Input: part model. Units: mm. Frame: model coordinates. Face numbers are marked on the shaded views. Give positions to 0.01 mm unless a question says otherwise; leave off trailing zeros. Write each loop counter-clockwise with the first axis right and the second up, starting at its lowest first coordinate (ties: lowest second). Pieces come first, ordered by that corner, then holes. Notation, with made-up numbers: (45.25, -10.5) - (54.25, -10.5) arc R12 ccw to (54.25, 6.5) - close; hole circle Ø7 at (83.5, 70). An arc over 180 degrees is marked (long way). Answer as CSV lines item,"result". Start each with the question number.
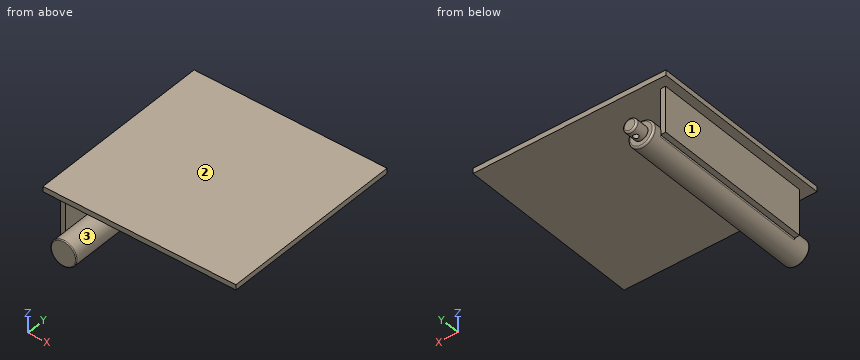
from build123d import *

# Parameters (mm, degrees)
SKETCH_1_W               = 110
SKETCH_1_H               = 106
EXTRUDE_1_DEPTH          = 3
SKETCH_2_W               = 3
SKETCH_2_H               = 94
EXTRUDE_2_DEPTH          = 38
EXTRUDE_3_DEPTH          = 5
EXTRUDE_3_DEPTH_BACK     = 104.122011
SKETCH_4_R               = 7.35
SKETCH_5_R               = 3.95
EXTRUDE_4_DEPTH          = 8
FILLET_2_R               = 1
CUT_EXTRUDE_1_DEPTH      = 155.044806793
CUT_EXTRUDE_1_DEPTH_BACK = 155.044806793
SKETCH_9_R               = 1.5
FILLET_3_R               = 0.5
SKETCH_11_W              = 3
SKETCH_11_H              = 94
CUT_EXTRUDE_3_DEPTH      = 12


with BuildPart() as part:
    # 草图1 → 凸台-拉伸1 (new body)
    with BuildSketch(Plane.XY):
        with Locations((55, 43)):
            Rectangle(SKETCH_1_W, SKETCH_1_H)
    extrude(amount=EXTRUDE_1_DEPTH)

    # 草图2 → 凸台-拉伸2 (add)
    with BuildSketch(Plane(origin=(0, 0, 0), x_dir=(-1, 0, 0), z_dir=(0, 0, -1))):
        with Locations((-6.5, 43)):
            Rectangle(SKETCH_2_W, SKETCH_2_H)
    extrude(amount=EXTRUDE_2_DEPTH)

    # 草图4 → 凸台-拉伸3 (add, two sides: drawn at the far end of the back side and taken through both)
    with BuildSketch(Plane(origin=(0, 90, 0), x_dir=(1, 0, 0), z_dir=(0, 1, 0)).offset(-EXTRUDE_3_DEPTH_BACK)):
        with Locations(Location((15, 25, 0), (0, 0, 270))):
            Circle(SKETCH_4_R)
    extrude(amount=EXTRUDE_3_DEPTH + EXTRUDE_3_DEPTH_BACK)

    # 草图5 → 凸台-拉伸4 (add)
    with BuildSketch(Plane(origin=(0, 95, 0), x_dir=(1, 0, 0), z_dir=(0, 1, 0))):
        with Locations(Location((15, 25, 0), (0, 0, 270))):
            Circle(SKETCH_5_R)
    extrude(amount=EXTRUDE_4_DEPTH)

    # 圆角2
    fillet_2_edges = [part.edges().sort_by_distance(p)[0] for p in [
        (15, 95, -32.35),
        (15, 103, -28.95),
    ]]
    fillet(fillet_2_edges, radius=FILLET_2_R)

    # 草图9 → 切除-拉伸1 (cut, two sides: drawn at the far end of the back side and taken through both)
    with BuildSketch(Plane(origin=(0, 0, -28.95), x_dir=(-1, 0, 0), z_dir=(0, 0, -1)).offset(-CUT_EXTRUDE_1_DEPTH_BACK)):
        with Locations(Location((-15, 98.677988735, 0), (0, 0, 90.000000013))):
            Circle(SKETCH_9_R)
    extrude(amount=CUT_EXTRUDE_1_DEPTH + CUT_EXTRUDE_1_DEPTH_BACK, mode=Mode.SUBTRACT)

    # 圆角3
    fillet_3_edges = [part.edges().sort_by_distance(p)[0] for p in [
        (15, -14.122011, -32.35),
    ]]
    fillet(fillet_3_edges, radius=FILLET_3_R)

    # 草图11 → 切除-拉伸3 (cut)
    with BuildSketch(Plane(origin=(0, 0, -38), x_dir=(-1, 0, 0), z_dir=(0, 0, -1))):
        with Locations((-6.5, 43)):
            Rectangle(SKETCH_11_W, SKETCH_11_H)
    extrude(amount=-CUT_EXTRUDE_3_DEPTH, mode=Mode.SUBTRACT)


solid = part.part
1) Contact query for flat-ended pins moving along their axis: P1, Ø1, axis at x = 68.5, y = 43.5, coming from the -Z side; P2, Ø1.5, axis at y = 2.5, z = -23.5, coming from the +X side; P3, Ø1.5, axis at x = 7, y = 36, coming from the -Z side. Output: stop coordinate, or through.
2) Cut plane B-B on y = 30. Output: boundary loops of the cut face in (x, z).
3) Pull-direction query (Z, two-part tool) for the marked faces 1, 2 and 3; classes: +Z half, -Z half, draft (parallel to the pull), parting line (faces both ways), or undercut.
4) Cut plane C-C on z = -10. Output: boundary loops of the cut face in (x, y), and give its area (3 significant figures).
5) Material intervals for line 1 (Z direction, x = 38.5, y = 72.5); line 2 (Z direction, x = 18.5, y = 94); line 3 (X direction, y = 85, z = -4), sorted ascending. Write a range as from..to.
6) Cut plane D-D on x = 90. Output: boundary loops of the cut face in (y, z).
7) Cut plane A-A on x = 15. Output: boundary loops of the cut face in (y, z), and give its area (3 significant figures).
Numbers:
1,P1,"stops at z = 0"
1,P2,"stops at x = 22.31"
1,P3,"stops at z = -26"
2,outline,"(0, 0) - (5, 0) - (5, -26) - (8, -26) - (8, -27.24) arc R7.35 ccw (long way) to (8, -22.76) - (8, 0) - (110, 0) - (110, 3) - (0, 3) - close"
3,face 1,"draft"
3,face 2,"+Z half"
3,face 3,"undercut"
4,outline,"(5, -4) - (8, -4) - (8, 90) - (5, 90) - close"
4,area,"282 mm²"
5,line 1,"z = 0..3"
5,line 2,"z = -31.46..-18.54, 0..3"
5,line 3,"x = 5..8"
6,outline,"(-10, 0) - (96, 0) - (96, 3) - (-10, 3) - close"
7,outline,"(-14.12, -31.85) arc R0.5 ccw to (-13.62, -32.35) - (94, -32.35) arc R1 ccw to (95, -31.35) - (95, -28.95) - (97.18, -28.95) - (97.18, -21.05) - (95, -21.05) - (95, -18.65) arc R1 ccw to (94, -17.65) - (-13.62, -17.65) arc R0.5 ccw to (-14.12, -18.15) - close; (-10, 0) - (96, 0) - (96, 3) - (-10, 3) - close; (100.18, -28.95) - (102, -28.95) arc R1 ccw to (103, -27.95) - (103, -22.05) arc R1 ccw to (102, -21.05) - (100.18, -21.05) - close"
7,area,"1,960 mm²"
